Can you work these out from the model? Positions are in its coordinate system, mm. A direction names the side the tool comes from. Give positions to 0.01 mm unless a question says otherwise; leave off trailing zeros. Order: outer loops, then holes, each group sorted by start corner. A loop starts at its lowest first (then second) coordinate and runs counter-clockwise, first axis right, second up. Notation, with made-up numbers: M 17,35 L 53,35 A17 cw 53,59 Z; hole C 65,70 d5. An arc over 180 degrees is marked long. One line per question, with ' | ' between items. Start each with the question number.
1) Thinking about a two-plate mould opening in X: for faces 1 (the cylindrical face through (-10.648, -1.232, -13.887)), 2 (the cylindrical face through (13.066, 1.268, 17.7)), 3 (the cylindrical face through (-20.525, 1.268, 0.474)), which applies, +X half, -X half, draft (parallel to the pull), parting line (faces both ways), or undercut?
2) If we section it at B-B, the plane x = -23.5: Please give me the cut outline in (y, z).
3) If we section it at C-C, the plane y = 1: State how many separate pieces and enclosed holes the cut face has, plus the area to 3 significant figures.
4) For faces 4 (the cylindrical face through (-19.598, 1.268, 42.052)), 5 (the cylindrical face through (-10.648, 3.486, -13.887)), which set-ups out of +Z, -Z, +X, -X, +Y, -Y let a thin tool reach every point of the face, with its end or its side?
5) Please list where these lines run through material, in increasing order: line 1 along X through (y, z) = (4.25, 0) (3 decimals); line 2 along Z through (x, y) = (8, 1.25); line 3 along Y through (x, z) = (13.5, 12). Write a range as [from, to].
6) I'm going to push flat-ended pins straight in: pin 1 Ø17.5 at (x, z) = (-21.25, -36.81) entering from -Y; pin 2 Ø3.5 at (x, z) = (0, 0) entering from +Y; pin 3 Ø3 at (x, y) = (15, 2.5) entering from +Z. Where does each tip first touch, or does it pass through?
7) If we section it at A-A, the plane z = 0: Please give me the cut outline in (x, y) (3 decimals), plus the area to 3 significant figures.
```python
from build123d import *

# Parameters (mm, degrees)
SKETCH1_W                 = 100
SKETCH1_H                 = 100
BOSS_EXTRUDE1_DEPTH       = 2.5
SKETCH2_W                 = 100
SKETCH2_H                 = 100
SKETCH2_R                 = 5.5
CUT_EXTRUDE1_DEPTH        = 10
CUT_EXTRUDE3_DEPTH        = 10
SKETCH6_R                 = 17.5
BOSS_EXTRUDE11_DEPTH      = 2
BOSS_EXTRUDE11_DEPTH_BACK = 5
SKETCH7_R                 = 1.425
CUT_EXTRUDE4_DEPTH        = 56.337685614


with BuildPart() as part:
    # Sketch1 → Boss-Extrude1 (new body)
    with BuildSketch(Plane(origin=(0, 0, 0), x_dir=(1, 0, 0), z_dir=(0, 1, 0))):
        Rectangle(SKETCH1_W, SKETCH1_H)
    extrude(amount=BOSS_EXTRUDE1_DEPTH)

    # Sketch2 → Cut-Extrude1 (cut)
    with BuildSketch(Plane(origin=(0, 2.5, 0), x_dir=(1, 0, 0), z_dir=(0, 1, 0))):
        Rectangle(SKETCH2_W, SKETCH2_H)
        with BuildLine():
            ThreePointArc((-29.074945731, -32.359707621), (-20.523161881, 0), (-29.074945731, 32.359707621))
            ThreePointArc((-29.074945731, 32.359707621), (-24.454355603, 45.216317777), (-12.450207096, 38.693841525))
            add(Edge.make_bspline(
                [(-12.450207096, 38.693841525), (0, -19.342739332), (12.450207096, 38.693841525)],
                knots=[5.128046308, 5.128046308, 5.128046308, 7.438324307, 7.438324307, 7.438324307], degree=2, weights=[1, 0.403791374, 1]))
            ThreePointArc((12.450207096, 38.693841525), (24.454355603, 45.216317777), (29.074945731, 32.359707621))
            ThreePointArc((29.074945731, 32.359707621), (20.523161881, 0), (29.074945731, -32.359707621))
            ThreePointArc((29.074945731, -32.359707621), (24.454355603, -45.216317777), (12.450207096, -38.693841525))
            add(Edge.make_bspline(
                [(12.450207096, -38.693841525), (0, 19.342739332), (-12.450207096, -38.693841525)],
                knots=[5.128046308, 5.128046308, 5.128046308, 7.438324307, 7.438324307, 7.438324307], degree=2, weights=[1, 0.403791374, 1]))
            ThreePointArc((-12.450207096, -38.693841525), (-24.454355603, -45.216317777), (-29.074945731, -32.359707621))
        make_face(mode=Mode.SUBTRACT)
        with Locations(Location((-21.25, 36.806079661, 0), (0, 0, 270))):
            Circle(SKETCH2_R)
        with Locations(Location((-21.25, -36.806079661, 0), (0, 0, 270))):
            Circle(SKETCH2_R)
        with Locations(Location((21.25, -36.806079661, 0), (0, 0, 270))):
            Circle(SKETCH2_R)
        with Locations(Location((21.25, 36.806079661, 0), (0, 0, 270))):
            Circle(SKETCH2_R)
    extrude(amount=-CUT_EXTRUDE1_DEPTH, mode=Mode.SUBTRACT)

    # Sketch4 → Cut-Extrude3 (cut)
    with BuildSketch(Plane(origin=(0, 2.5, 0), x_dir=(1, 0, 0), z_dir=(0, 1, 0))):
        with BuildLine():
            ThreePointArc((-17.749489284, -12.998293356), (-13.140045691, -17.64480658), (-7.367625104, -20.729643034))
            add(Edge.make_bspline(
                [(-7.367625104, -20.729643034), (-7.747241798, -21.030061446), (-8.114529726, -21.350348356), (-9.247106431, -22.428016295), (-9.96747496, -23.25295704), (-11.975526868, -25.945450431), (-13.113170007, -28.031524091), (-14.161311212, -30.568863064), (-14.254109179, -30.800153833), (-14.345065296, -31.033569225)],
                knots=[0.658936879, 0.658936879, 0.658936879, 0.658936879, 0.6875, 0.6875, 0.75, 0.75, 0.875, 0.875, 0.887405876, 0.887405876, 0.887405876, 0.887405876], degree=3))
            ThreePointArc((-14.345065296, -31.033569225), (-17.949067849, -28.433275654), (-22.357942029, -27.874536431))
            add(Edge.make_bspline(
                [(-17.749489284, -12.998293356), (-18.730013182, -18.148505445), (-20.279042278, -23.126345909), (-22.357942029, -27.874536431)],
                knots=[0.6784999, 0.6784999, 0.6784999, 0.6784999, 0.896036051, 0.896036051, 0.896036051, 0.896036051], degree=3, weights=[0.94303917, 0.94979881, 0.960677405, 0.975674954]))
        make_face()
        with BuildLine():
            ThreePointArc((7.367625104, -20.729643034), (13.140045691, -17.64480658), (17.749489284, -12.998293356))
            add(Edge.make_bspline(
                [(22.357942029, -27.874536431), (20.279042278, -23.126345909), (18.730013182, -18.148505445), (17.749489284, -12.998293356)],
                knots=[0.103963949, 0.103963949, 0.103963949, 0.103963949, 0.3215001, 0.3215001, 0.3215001, 0.3215001], degree=3, weights=[0.975674954, 0.960677405, 0.94979881, 0.94303917]))
            ThreePointArc((22.357942029, -27.874536431), (17.949067849, -28.433275654), (14.345065296, -31.033569225))
            add(Edge.make_bspline(
                [(14.345065296, -31.033569225), (14.254109179, -30.800153832), (14.161311212, -30.568863064), (13.113170007, -28.031524091), (11.975526868, -25.945450431), (9.96747496, -23.25295704), (9.247106431, -22.428016295), (8.114529726, -21.350348356), (7.747241798, -21.030061447), (7.367625104, -20.729643034)],
                knots=[0.112594124, 0.112594124, 0.112594124, 0.112594124, 0.125, 0.125, 0.25, 0.25, 0.3125, 0.3125, 0.341063121, 0.341063121, 0.341063121, 0.341063121], degree=3))
        make_face()
        with BuildLine():
            ThreePointArc((14.345065296, 31.033569225), (17.949067849, 28.433275654), (22.357942029, 27.874536431))
            add(Edge.make_bspline(
                [(17.749489284, 12.998293356), (18.730013182, 18.148505445), (20.279042278, 23.126345909), (22.357942029, 27.874536431)],
                knots=[0.6784999, 0.6784999, 0.6784999, 0.6784999, 0.896036051, 0.896036051, 0.896036051, 0.896036051], degree=3, weights=[0.94303917, 0.94979881, 0.960677405, 0.975674954]))
            ThreePointArc((17.749489284, 12.998293356), (13.140045691, 17.64480658), (7.367625104, 20.729643034))
            add(Edge.make_bspline(
                [(7.367625104, 20.729643034), (7.747241798, 21.030061446), (8.114529726, 21.350348356), (9.247106431, 22.428016295), (9.96747496, 23.25295704), (11.975526868, 25.945450431), (13.113170007, 28.031524091), (14.161311212, 30.568863064), (14.254109179, 30.800153833), (14.345065296, 31.033569225)],
                knots=[0.658936879, 0.658936879, 0.658936879, 0.658936879, 0.6875, 0.6875, 0.75, 0.75, 0.875, 0.875, 0.887405876, 0.887405876, 0.887405876, 0.887405876], degree=3))
        make_face()
        with BuildLine():
            ThreePointArc((-14.345065296, 31.033569225), (-17.949067849, 28.433275654), (-22.357942029, 27.874536431))
            add(Edge.make_bspline(
                [(-22.357942029, 27.874536431), (-20.279042278, 23.126345909), (-18.730013182, 18.148505445), (-17.749489284, 12.998293356)],
                knots=[0.103963949, 0.103963949, 0.103963949, 0.103963949, 0.3215001, 0.3215001, 0.3215001, 0.3215001], degree=3, weights=[0.975674954, 0.960677405, 0.94979881, 0.94303917]))
            ThreePointArc((-17.749489284, 12.998293356), (-13.140045691, 17.64480658), (-7.367625104, 20.729643034))
            add(Edge.make_bspline(
                [(-14.345065296, 31.033569225), (-14.254109179, 30.800153832), (-14.161311212, 30.568863064), (-13.113170007, 28.031524091), (-11.975526868, 25.945450431), (-9.96747496, 23.25295704), (-9.247106431, 22.428016295), (-8.114529726, 21.350348356), (-7.747241798, 21.030061447), (-7.367625104, 20.729643034)],
                knots=[0.112594124, 0.112594124, 0.112594124, 0.112594124, 0.125, 0.125, 0.25, 0.25, 0.3125, 0.3125, 0.341063121, 0.341063121, 0.341063121, 0.341063121], degree=3))
        make_face()
    extrude(amount=-CUT_EXTRUDE3_DEPTH, mode=Mode.SUBTRACT)

    # Sketch6 → Boss-Extrude11 (add, two sides)
    with BuildSketch(Plane(origin=(0, 2.5, 0), x_dir=(1, 0, 0), z_dir=(0, 1, 0))) as boss_extrude11_sk:
        with Locations(Location((0, 0, 0), (0, 0, 270))):
            Circle(SKETCH6_R)
    extrude(amount=BOSS_EXTRUDE11_DEPTH)
    extrude(boss_extrude11_sk.sketch, amount=-BOSS_EXTRUDE11_DEPTH_BACK)

    # Sketch7 → Cut-Extrude4 (cut, through all)
    with BuildSketch(Plane(origin=(0, 4.5, 0), x_dir=(1, 0, 0), z_dir=(0, 1, 0))):
        with Locations(Location((0, 0, 0), (0, 0, 270))):
            Circle(SKETCH7_R)
    extrude(amount=-CUT_EXTRUDE4_DEPTH, mode=Mode.SUBTRACT)


solid = part.part
```
Results found:
1) face 1: parting line | face 2: undercut | face 3: -X half
2) outline: M 0,-45.52 L 2.5,-45.52 L 2.5,-41.82 L 0,-41.82 Z; M 0,-31.79 L 2.5,-31.79 L 2.5,-19.52 L 0,-19.52 Z; M 0,19.52 L 2.5,19.52 L 2.5,31.79 L 0,31.79 Z; M 0,41.82 L 2.5,41.82 L 2.5,45.52 L 0,45.52 Z
3) separate pieces: 1 | enclosed holes: 9 | area: 2,680 mm²
4) face 4: +Y, -Y | face 5: +Y
5) line 1: x = [-17.5, -1.425], [1.425, 17.5] | line 2: z = [-27.35, -21.26], [-20.49, 20.49], [21.26, 27.35] | line 3: y = [0, 2.5]
6) pin 1: stops at y = 0 | pin 2: stops at y = 4.5 | pin 3: stops at z = 44.45
7) outline: M -20.523,0 L -17.5,0 L -17.5,-2.5 L -1.425,-2.5 L -1.425,4.5 L -17.5,4.5 L -17.5,2.5 L -20.523,2.5 Z; M 1.425,-2.5 L 17.5,-2.5 L 17.5,0 L 20.523,0 L 20.523,2.5 L 17.5,2.5 L 17.5,4.5 L 1.425,4.5 Z | area: 240 mm²
